Verification items for the finished model (mm, model axes). A direction names the side the tool comes from. Give positions to 0.01 mm unless a question says otherwise; leave off trailing zeros. Write each loop counter-clockwise with the first axis right and the second up, starting at its lowest first coordinate (ties: lowest second). Pieces come first, ordered by that corner, then holes.
from build123d import *

# Parameters (mm, degrees)
F0_W     = 100
F0_H     = 100
F0_R     = 25
F1_DEPTH = 100
F2_R     = 23.481347
F3_DEPTH = 50
F4_W     = 50
F4_H     = 50
F5_DEPTH = 25
F6_R     = 34.48111
F7_DEPTH = 25
F8_R     = 10.324712
F9_DEPTH = 89


with BuildPart() as f1:
    # F0 (on Top) → F1 (new body)
    with BuildSketch(Plane.XY):
        with Locations((1.244521, -3.481347)):
            Rectangle(F0_W, F0_H)
        Circle(F0_R, mode=Mode.SUBTRACT)
    extrude(amount=F1_DEPTH)

    # F2 (on face) → F3 (cut)
    with BuildSketch(Plane.XY.offset(100)):
        with Locations((0, -53.481347)):
            Circle(F2_R)
    extrude(amount=-F3_DEPTH, mode=Mode.SUBTRACT)

    # F4 (on face) → F5 (join)
    with BuildSketch(Plane(origin=(-48.755479, 0, 0), x_dir=(0, -1, 0), z_dir=(-1, 0, 0))):
        with Locations((2.66633, 44.168345)):
            Rectangle(F4_W, F4_H)
    extrude(amount=F5_DEPTH)

    # F6 (on Top) → F7 (join)
    with BuildSketch(Plane.XY):
        with Locations((55.731513, -54.766722)):
            Circle(F6_R)
    extrude(amount=F7_DEPTH)

    # F8 (on face) → F9 (join)
    with BuildSketch(Plane.XY.offset(100)):
        with Locations((35.525516, 29.389268)):
            Circle(F8_R)
    extrude(amount=F9_DEPTH)


solid = f1.part
Item 1: Scan lines: line 1 along Z through (x, y) = (-45, -23); line 2 along Y through (x, z) = (-63.5, 57); line 3 along Y through (x, z) = (0, 43). Record each from-to range of solid material in increasing order.
Answer key:
line 1: z = 0 to 100
line 2: y = -27.67 to 22.33
line 3: y = -53.48 to -25, 25 to 46.52
Item 2: Sectioned sample at D-D on z = 171. Record the cut outline in (x, y), then the cut area to 3 significant figures.
Answer key:
outline: circle Ø20.65 at (35.53, 29.39)
area: 335 mm2
Item 3: Release check for a two-part mould opening along Y. For faces 1 (the face through (23.846, 7.509, 49.3)), 2 (the face through (-61, -2, 19.168)), 3 (the face through (45.06, 25.43, 143.88)) record: released by +Y, released by -Y, zero draft, split by the parting line, or undercut.
Answer key:
face 1: undercut
face 2: zero draft
face 3: split by the parting line
Item 4: Sectioned sample at C-C on x = -63. Record the cut outline in (y, z).
Answer key:
outline: (-27.67, 19.17) - (22.33, 19.17) - (22.33, 69.17) - (-27.67, 69.17) - close
Item 5: Depth check by flat-ended pin: pin 1 (20 mm diameter, centred on x = -60.5, z = 47, fed in from +Y); pin 2 (6 mm diameter, centred on y = -45, z = 27, fed in from -X); pin 3 (20 mm diameter, centred on x = -60, y = -10, fed in from -Z); pin 4 (5 mm diameter, centred on x = -12.5, y = -57, fed in from +Z). Enter the tip coordinate at first touch or a pass-through.
Answer key:
pin 1: stops at y = 22.33
pin 2: stops at x = -48.76
pin 3: stops at z = 19.17
pin 4: passes through
Item 6: Set-up check for faces 4 (the face through (-61, -27.666, 44)), 5 (the face through (-61, 22.334, 44)), 6 (the face through (0, -44, 50)): record each of +Z, -Z, +X, -X, +Y, -Y from which the full face is reachable in a straight line by a thin tool's end or side.
Answer key:
face 4: +Z, -Z, -X, -Y
face 5: +Z, -Z, -X, +Y
face 6: +Z, -Y
Item 7: Sectioned sample at B-B on x = 0. Record the cut outline in (y, z), then the cut area to 3 significant figures.
Answer key:
outline: (-53.48, 0) - (-25, 0) - (-25, 100) - (-30, 100) - (-30, 50) - (-53.48, 50) - close; (25, 0) - (46.52, 0) - (46.52, 100) - (25, 100) - close
area: 3,830 mm2
Item 8: Sectioned sample at A-A on y = 0. Record the cut outline in (x, z), then the cut area to 3 significant figures.
Answer key:
outline: (-73.76, 19.17) - (-48.76, 19.17) - (-48.76, 0) - (-25, 0) - (-25, 100) - (-48.76, 100) - (-48.76, 69.17) - (-73.76, 69.17) - close; (25, 0) - (51.24, 0) - (51.24, 100) - (25, 100) - close
area: 6,250 mm2
